Work out the finished part from the listing and answer in its coordinate system (mm). Face numbers are marked on the shaded views. A direction names the side the tool comes from. Round coordinates to 2 decimals unless told otherwise and drop trailing zeros. Loops run counter-clockwise (first coordinate to the right, second up) from the corner with the lowest first, then second, coordinate; pieces in that order, holes last.
```python
from build123d import *

# Parameters (mm, degrees)
SKETCH1_R           = 80
SKETCH1_R_2         = 5.2
BOSS_EXTRUDE1_DEPTH = 2
SKETCH2_R           = 2.5
CUT_EXTRUDE1_DEPTH  = 114.154761279
SKETCH3_R           = 13.5
SKETCH3_R_2         = 5.2
BOSS_EXTRUDE2_DEPTH = 8
SKETCH4_R           = 13.5
SKETCH4_R_2         = 11.2
BOSS_EXTRUDE3_DEPTH = 8


with BuildPart() as part:
    # Sketch1 → Boss-Extrude1 (new body)
    with BuildSketch(Plane(origin=(0, 0, 0), x_dir=(1, 0, 0), z_dir=(0, 1, 0))):
        with Locations(Location((0, 0, 0), (0, 0, 270))):
            Circle(SKETCH1_R)
        with Locations(Location((0, 0, 0), (0, 0, 270))):
            Circle(SKETCH1_R_2, mode=Mode.SUBTRACT)
    extrude(amount=BOSS_EXTRUDE1_DEPTH)

    # Sketch2 → Cut-Extrude1 (cut, through all)
    with BuildSketch(Plane(origin=(0, 2, 0), x_dir=(1, 0, 0), z_dir=(0, 1, 0))):
        with Locations(Location((0, 73, 0), (0, 0, 270))):
            Circle(SKETCH2_R)
        with Locations(Location((73, 0, 0), (0, 0, 270))):
            Circle(SKETCH2_R)
        with Locations(Location((0, -73, 0), (0, 0, 270))):
            Circle(SKETCH2_R)
        with Locations(Location((-73, 0, 0), (0, 0, 270))):
            Circle(SKETCH2_R)
    extrude(amount=-CUT_EXTRUDE1_DEPTH, mode=Mode.SUBTRACT)

    # Sketch3 → Boss-Extrude2 (add)
    with BuildSketch(Plane(origin=(0, 2, 0), x_dir=(1, 0, 0), z_dir=(0, 1, 0))):
        with Locations(Location((0, 0, 0), (0, 0, 270))):
            Circle(SKETCH3_R)
        with Locations(Location((0, 0, 0), (0, 0, 270))):
            Circle(SKETCH3_R_2, mode=Mode.SUBTRACT)
    extrude(amount=BOSS_EXTRUDE2_DEPTH)

    # Sketch4 → Boss-Extrude3 (add)
    with BuildSketch(Plane(origin=(0, 10, 0), x_dir=(1, 0, 0), z_dir=(0, 1, 0))):
        with Locations(Location((0, 0, 0), (0, 0, 270))):
            Circle(SKETCH4_R)
        with Locations(Location((0, 0, 0), (0, 0, 270))):
            Circle(SKETCH4_R_2, mode=Mode.SUBTRACT)
    extrude(amount=BOSS_EXTRUDE3_DEPTH)


solid = part.part
```
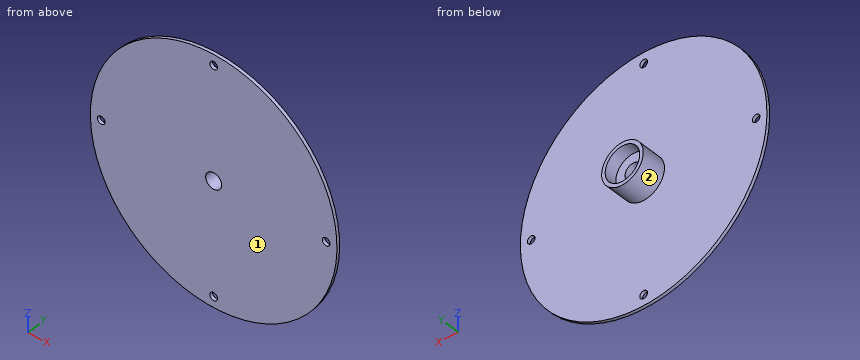
1. Find section C-C (x = -73). Write down the section's boundary in (y, z).
Answer key:
outline: (0, -32.73) - (2, -32.73) - (2, -2.5) - (0, -2.5) - close; (0, 2.5) - (2, 2.5) - (2, 32.73) - (0, 32.73) - close
2. Find section D-D (y = 12.5). Write down the section's boundary in (x, z), then the cut area to 3 significant figures.
Answer key:
outline: circle Ø27 at (0, 0); hole circle Ø22.4 at (0, 0)
area: 178 mm2
3. Find section A-A (x = 0). Write down the section's boundary in (y, z).
Answer key:
outline: (0, -80) - (2, -80) - (2, -75.5) - (0, -75.5) - close; (0, -70.5) - (2, -70.5) - (2, -13.5) - (18, -13.5) - (18, -11.2) - (10, -11.2) - (10, -5.2) - (0, -5.2) - close; (0, 5.2) - (10, 5.2) - (10, 11.2) - (18, 11.2) - (18, 13.5) - (2, 13.5) - (2, 70.5) - (0, 70.5) - close; (0, 75.5) - (2, 75.5) - (2, 80) - (0, 80) - close
4. Consider probe 1 along X at (y, z) = (0.9, 0); probe 2 along Y at (x, z) = (-14, -19); probe 3 along X at (y, z) = (1.3, 73). Determine where each line is inside the solid, lowest interval first.
Answer key:
probe 1: x = -80 to -75.5, -70.5 to -5.2, 5.2 to 70.5, 75.5 to 80
probe 2: y = 0 to 2
probe 3: x = -32.73 to -2.5, 2.5 to 32.73
5. Find section B-B (z = 73). Write down the section's boundary in (x, y), then the cut area to 3 significant figures.
Answer key:
outline: (-32.73, 0) - (-2.5, 0) - (-2.5, 2) - (-32.73, 2) - close; (2.5, 0) - (32.73, 0) - (32.73, 2) - (2.5, 2) - close
area: 121 mm2
6. Which of the six approach directions +Z, -Z, +X, -X, +Y, -Y give full straight-line access (tool end or side, diameter ignored) to the marked faces 1 and 2?
Answer key:
face 1: +Z, -Z, +X, -X, -Y
face 2: +Y
7. Given pin 1 (6 mm diameter, centred on y = 2.5, z = -43, fed in from +X); pin 2 (6 mm diameter, centred on x = -73, z = 0, fed in from +Y); pin 3 (10 mm diameter, centred on y = 6, z = -15.5, fed in from -X); pin 4 (3 mm diameter, centred on x = 0, z = -73, fed in from -Y), each flat-ended and moving along its own axis, determine where each tip first touches the part or whether it passes through.
Answer key:
pin 1: stops at x = 69.26
pin 2: stops at y = 2
pin 3: stops at x = -79.02
pin 4: passes through
